```python
from build123d import *

# Parameters (mm, degrees)
SKETCH1_W               = 44.958
SKETCH1_H               = 304.8
BOSS_EXTRUDE1_DEPTH     = 3.175
BOSS_EXTRUDE2_DEPTH     = 3.175
SKETCH3_W               = 123.825
SKETCH3_H               = 6.35
BOSS_EXTRUDE3_DEPTH     = 41.783
SKETCH8_W               = 3.175
SKETCH8_H               = 213.451350416
CUT_EXTRUDE4_DEPTH      = 1
CUT_EXTRUDE4_DEPTH_BACK = 131.175
SKETCH6_W               = 3.175
SKETCH6_H               = 12.7
CUT_EXTRUDE5_DEPTH      = 3.175
SKETCH4_3_W             = 6.35
SKETCH4_3_H             = 15.875
SKETCH4_3_H_2           = 5.588
SKETCH4_3_H_3           = 7.112
CUT_EXTRUDE6_DEPTH      = 6.35
CUT_EXTRUDE7_DEPTH      = 4.175


with BuildPart() as part:
    # Sketch1 → Boss-Extrude1 (new body)
    with BuildSketch(Plane.XY):
        with Locations((-6.477, 3.048)):
            Rectangle(SKETCH1_W, SKETCH1_H)
        with BuildLine():
            Line((-3.302, 133.858), (-3.302, -143.002))
            Line((-3.302, -143.002), (3.302, -143.002))
            Line((3.302, -143.002), (3.302, 143.002))
            Line((3.302, 143.002), (-16.256, 143.002))
            Line((-16.256, 143.002), (-16.256, 136.398))
            Line((-16.256, 136.398), (-5.842, 136.398))
            ThreePointArc((-5.842, 136.398), (-4.045948776, 135.654051224), (-3.302, 133.858))
        make_face(mode=Mode.SUBTRACT)
    extrude(amount=BOSS_EXTRUDE1_DEPTH)

    # Sketch2 → Boss-Extrude2 (add)
    with BuildSketch(Plane(origin=(16.002, 0, 0), x_dir=(0, 0, -1), z_dir=(1, 0, 0))):
        Polygon((123.825, -47.752), (-3.175, -47.752), (-3.175, -149.352), (123.825, -149.352), (123.825, -136.652), (127, -136.652), (127, -119.718666667), (123.825, -119.718666667), (123.825, -107.018666667), (127, -107.018666667), (127, -90.085333333), (123.825, -90.085333333), (123.825, -77.385333333), (127, -77.385333333), (127, -60.452), (123.825, -60.452), align=None)
        with BuildLine():
            ThreePointArc((11.9, -106.092), (10.4, -107.592), (8.9, -106.092))
            Line((8.9, -106.092), (8.9, -101.012))
            ThreePointArc((8.9, -101.012), (10.4, -99.512), (11.9, -101.012))
            Line((11.9, -101.012), (11.9, -106.092))
        make_face(mode=Mode.SUBTRACT)
        with BuildLine():
            ThreePointArc((60.9, -106.092), (59.4, -107.592), (57.9, -106.092))
            Line((57.9, -106.092), (57.9, -101.012))
            ThreePointArc((57.9, -101.012), (59.4, -99.512), (60.9, -101.012))
            Line((60.9, -101.012), (60.9, -106.092))
        make_face(mode=Mode.SUBTRACT)
        with BuildLine():
            Line((8.9, -96.092), (8.9, -91.012))
            ThreePointArc((8.9, -91.012), (10.4, -89.512), (11.9, -91.012))
            Line((11.9, -91.012), (11.9, -96.092))
            ThreePointArc((11.9, -96.092), (10.4, -97.592), (8.9, -96.092))
        make_face(mode=Mode.SUBTRACT)
        with BuildLine():
            ThreePointArc((36.4, -101.092), (25.4, -112.092), (14.4, -101.092))
            Line((14.4, -101.092), (14.4, -96.012))
            ThreePointArc((14.4, -96.012), (25.4, -85.012), (36.4, -96.012))
            Line((36.4, -96.012), (36.4, -101.092))
        make_face(mode=Mode.SUBTRACT)
        with BuildLine():
            ThreePointArc((57.9, -91.012), (59.4, -89.512), (60.9, -91.012))
            Line((60.9, -91.012), (60.9, -96.092))
            ThreePointArc((60.9, -96.092), (59.4, -97.592), (57.9, -96.092))
            Line((57.9, -96.092), (57.9, -91.012))
        make_face(mode=Mode.SUBTRACT)
    extrude(amount=-BOSS_EXTRUDE2_DEPTH)

    # Sketch3 → Boss-Extrude3 (add)
    with BuildSketch(Plane.ZY.offset(-12.827)):
        with Locations((-61.9125, -146.177)):
            Rectangle(SKETCH3_W, SKETCH3_H)
    extrude(amount=BOSS_EXTRUDE3_DEPTH)

    # Sketch8 → Cut-Extrude4 (cut, two sides)
    with BuildSketch(Plane.XY.offset(3.175)) as cut_extrude4_sk:
        Polygon((-28.956, -149.352), (12.827, -149.352), (12.827, -47.752), (12.827, 155.448), (-28.956, 155.448), align=None)
        with BuildLine():
            Line((-16.256, 136.398), (-16.256, 143.002))
            Line((-16.256, 143.002), (3.302, 143.002))
            Line((3.302, 143.002), (3.302, -143.002))
            Line((3.302, -143.002), (-3.302, -143.002))
            Line((-3.302, -143.002), (-3.302, 133.858))
            ThreePointArc((-3.302, 133.858), (-4.045948776, 135.654051224), (-5.842, 136.398))
            Line((-5.842, 136.398), (-16.256, 136.398))
        make_face(mode=Mode.SUBTRACT)
        Polygon((-54.223542679, -149.352), (-28.956, -149.352), (-28.956, 155.448), (12.827, 155.448), (12.827, 165.699350416), (-54.223542679, 165.699350416), align=None)
        with Locations((14.4145, 58.973675208)):
            Rectangle(SKETCH8_W, SKETCH8_H)
    extrude(amount=CUT_EXTRUDE4_DEPTH, mode=Mode.SUBTRACT)
    extrude(cut_extrude4_sk.sketch, amount=-CUT_EXTRUDE4_DEPTH_BACK, mode=Mode.SUBTRACT)

    # Sketch6 → Cut-Extrude5 (cut)
    with BuildSketch(Plane.XY.offset(3.175)):
        with Locations((14.4145, -54.102)):
            Rectangle(SKETCH6_W, SKETCH6_H)
        with Locations((14.4145, -83.735333333)):
            Rectangle(SKETCH6_W, SKETCH6_H)
        with Locations((14.4145, -113.368666667)):
            Rectangle(SKETCH6_W, SKETCH6_H)
        with Locations((14.4145, -143.002)):
            Rectangle(SKETCH6_W, SKETCH6_H)
    extrude(amount=-CUT_EXTRUDE5_DEPTH, mode=Mode.SUBTRACT)

    # Sketch4_3 → Cut-Extrude6 (cut)
    with BuildSketch(Plane.XZ.offset(149.352)):
        with Locations((12.827, -103.1875)):
            Rectangle(SKETCH4_3_W, SKETCH4_3_H)
        with Locations((12.827, -74.6125)):
            Rectangle(SKETCH4_3_W, SKETCH4_3_H)
        with Locations((12.827, -46.0375)):
            Rectangle(SKETCH4_3_W, SKETCH4_3_H)
        with Locations((12.827, -17.4625)):
            Rectangle(SKETCH4_3_W, SKETCH4_3_H)
        with Locations((12.827, 0.381)):
            Rectangle(SKETCH4_3_W, SKETCH4_3_H_2)
        with Locations((12.827, -5.969)):
            Rectangle(SKETCH4_3_W, SKETCH4_3_H_3)
    extrude(amount=-CUT_EXTRUDE6_DEPTH, mode=Mode.SUBTRACT)

    # Sketch9 → Cut-Extrude7 (cut, through all)
    with BuildSketch(Plane(origin=(16.002, 0, 0), x_dir=(0, 0, -1), z_dir=(1, 0, 0))):
        with BuildLine():
            ThreePointArc((7.197741164, -98.552), (12.777356982, -85.081615818), (26.247741164, -79.502))
            Line((26.247741164, -79.502), (13.547741164, -79.502))
            ThreePointArc((13.547741164, -79.502), (9.057613103, -81.361871939), (7.197741164, -85.852))
            Line((7.197741164, -85.852), (7.197741164, -98.552))
        make_face()
        with BuildLine():
            ThreePointArc((26.247741164, -117.602), (12.777356982, -112.022384182), (7.197741164, -98.552))
            Line((7.197741164, -98.552), (7.197741164, -111.252))
            ThreePointArc((7.197741164, -111.252), (9.057613103, -115.742128061), (13.547741164, -117.602))
            Line((13.547741164, -117.602), (26.247741164, -117.602))
        make_face()
        with BuildLine():
            Line((59.4, -79.502), (26.247741164, -79.502))
            ThreePointArc((26.247741164, -79.502), (16.074520569, -82.445849537), (9.045492178, -90.367555619))
            ThreePointArc((9.045492178, -90.367555619), (7.665419684, -94.356785058), (7.197741164, -98.552))
            ThreePointArc((7.197741164, -98.552), (7.665419676, -102.747214908), (9.045492148, -106.736444318))
            ThreePointArc((9.045492148, -106.736444318), (16.07452054, -114.658150444), (26.247741164, -117.602))
            Line((26.247741164, -117.602), (59.4, -117.602))
            ThreePointArc((59.4, -117.602), (78.45, -98.552), (59.4, -79.502))
        make_face()
        with BuildLine():
            ThreePointArc((11.9, -106.092), (10.73033182, -107.555174935), (9.045492148, -106.736444318))
            ThreePointArc((9.045492148, -106.736444318), (8.936825065, -106.42233182), (8.9, -106.092))
            Line((8.9, -106.092), (8.9, -101.012))
            ThreePointArc((8.9, -101.012), (10.4, -99.512), (11.9, -101.012))
            Line((11.9, -101.012), (11.9, -106.092))
        make_face(mode=Mode.SUBTRACT)
        with BuildLine():
            ThreePointArc((14.4, -96.012), (25.4, -85.012), (36.4, -96.012))
            Line((36.4, -96.012), (36.4, -101.092))
            ThreePointArc((36.4, -101.092), (25.4, -112.092), (14.4, -101.092))
            Line((14.4, -101.092), (14.4, -96.012))
        make_face(mode=Mode.SUBTRACT)
        with BuildLine():
            Line((60.9, -101.012), (60.9, -106.092))
            ThreePointArc((60.9, -106.092), (59.4, -107.592), (57.9, -106.092))
            Line((57.9, -106.092), (57.9, -101.012))
            ThreePointArc((57.9, -101.012), (59.4, -99.512), (60.9, -101.012))
        make_face(mode=Mode.SUBTRACT)
        with BuildLine():
            ThreePointArc((8.9, -91.012), (8.936825073, -90.681668146), (9.045492178, -90.367555619))
            ThreePointArc((9.045492178, -90.367555619), (10.730331854, -89.548825073), (11.9, -91.012))
            Line((11.9, -91.012), (11.9, -96.092))
            ThreePointArc((11.9, -96.092), (10.4, -97.592), (8.9, -96.092))
            Line((8.9, -96.092), (8.9, -91.012))
        make_face(mode=Mode.SUBTRACT)
        with BuildLine():
            Line((60.9, -91.012), (60.9, -96.092))
            ThreePointArc((60.9, -96.092), (59.4, -97.592), (57.9, -96.092))
            Line((57.9, -96.092), (57.9, -91.012))
            ThreePointArc((57.9, -91.012), (59.4, -89.512), (60.9, -91.012))
        make_face(mode=Mode.SUBTRACT)
    extrude(amount=-CUT_EXTRUDE7_DEPTH, mode=Mode.SUBTRACT)


solid = part.part
```
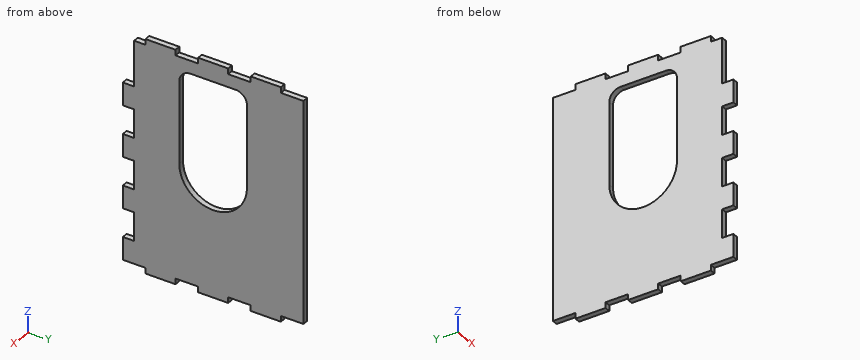
For this review, take the finished solid that the model builds, in its own axes (mm). Round coordinates to 2 decimals unless told otherwise and drop trailing zeros. Order: outer loops, then holes, each group sorted by start corner. A loop starts at its lowest first (then second) coordinate and runs counter-clockwise, first axis right, second up.
Q1. Insertion check: P1, Ø1.6, axis at x = 15, z = -73.5, coming from the -Y side; P2, Ø1, axis at x = 14.5, y = -114, coming from the +Z side; P3, Ø1.6, axis at x = 14.5, y = -146.5, coming from the +Z side. Each pin has a flat end and moves straight along its axis. Give the tip position at first contact, or say it passes through.
Findings below:
P1: stops at y = -143
P2: stops at z = 0
P3: stops at z = -25.4
Q2. We need section C-C, the plane z = -11. Give the boundary of the cut face in (x, y), plus the area to 3 significant figures.
Findings below:
outline: (12.83, -143) - (16, -143) - (16, -117.07) - (12.83, -117.07) - close; (12.83, -80.04) - (16, -80.04) - (16, -47.75) - (12.83, -47.75) - close
area: 185 mm2
Q3. Wall thickness on line 1 (Y direction, x = 14.1, z = -51.5); line 2 (Z direction, x = 14.6, y = -98) (3 decimals); line 3 (Y direction, x = 15.95, z = -105): over which ranges is each line inside the solid? List them lowest first.
Findings below:
line 1: y = -143 to -117.6, -79.5 to -47.75
line 2: z = -127 to -78.442, -7.198 to 3.175
line 3: y = -143 to -47.75
Q4. We need section B-B, the plane z = -108. Give the boundary of the cut face in (x, y).
Findings below:
outline: (12.83, -143) - (16, -143) - (16, -47.75) - (12.83, -47.75) - close
Q5. We need section A-A, the plane z = -45. Give the boundary of the cut face in (x, y).
Findings below:
outline: (12.83, -143) - (16, -143) - (16, -117.6) - (12.83, -117.6) - close; (12.83, -79.5) - (16, -79.5) - (16, -47.75) - (12.83, -47.75) - close
